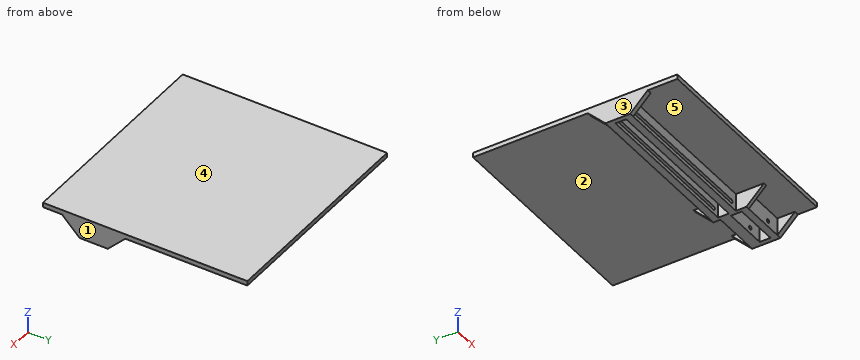
```python
from build123d import *

# Parameters (mm, degrees)
SKETCH_1_W          = 185
SKETCH_1_H          = 175
EXTRUDE_1_DEPTH     = 4
SKETCH_2_W          = 140
SKETCH_2_H          = 6
EXTRUDE_2_DEPTH     = 15
CUT_EXTRUDE_1_REACH = 210.987
SKETCH_4_W          = 45
SKETCH_4_H          = 9
SKETCH_4_H_2        = 6
EXTRUDE_5_DEPTH     = 15
SKETCH_7_W          = 185
SKETCH_7_H          = 4
EXTRUDE_6_DEPTH     = 40
SKETCH_6_W          = 185
SKETCH_6_H          = 4
CUT_EXTRUDE_3_DEPTH = 40
CUT_EXTRUDE_START   = -24.2
SKETCH_5_R          = 1.6
CUT_EXTRUDE_2_DEPTH = 24.2
EXTRUDE_7_DEPTH     = 3
EXTRUDE_8_DEPTH     = 4
EXTRUDE_9_DEPTH     = 4


with BuildPart() as part:
    # Sketch 1 → Extrude 1 (new body)
    with BuildSketch(Plane.XY):
        with Locations((21.366509782, 20.973731884)):
            Rectangle(SKETCH_1_W, SKETCH_1_H)
    extrude(amount=EXTRUDE_1_DEPTH)

    # Sketch 2 → Extrude 2 (add)
    with BuildSketch(Plane(origin=(0, 0, 0), x_dir=(-1, 0, 0), z_dir=(0, 0, -1))):
        with Locations((1.133490218, -63.126268116)):
            Rectangle(SKETCH_2_W, SKETCH_2_H)
        with Locations((1.133490218, -47.926268116)):
            Rectangle(SKETCH_2_W, SKETCH_2_H)
    extrude(amount=EXTRUDE_2_DEPTH)

    # Cut-Extrude 1: up to this face of the body (flat: up to its plane)
    cut_extrude_1_end = Plane(part.part.faces().sort_by_distance((-1.133490218, -44.926268116, -7.5))[0])
    # Sketch 3 → Cut-Extrude 1 (cut, up to the picked face)
    with BuildSketch(Plane.XZ.offset(66.126268116), mode=Mode.PRIVATE) as cut_extrude_1_sk1:
        with BuildLine():
            Line((-65.133490218, -8.4), (62.866509782, -8.4))
            ThreePointArc((62.866509782, -8.4), (64.466509782, -10), (62.866509782, -11.6))
            Line((62.866509782, -11.6), (-65.133490218, -11.6))
            ThreePointArc((-65.133490218, -11.6), (-66.733490218, -10), (-65.133490218, -8.4))
        make_face()
    cut_extrude_1_tool1 = split(extrude(cut_extrude_1_sk1.sketch, amount=-CUT_EXTRUDE_1_REACH, mode=Mode.PRIVATE), bisect_by=cut_extrude_1_end, keep=Keep.BOTH, mode=Mode.PRIVATE)
    add(cut_extrude_1_tool1.solids().sort_by(Axis((-1.13349, -66.126268, -10), (0, 1, 0)))[0], mode=Mode.SUBTRACT)

    # Sketch 4 → Extrude 5 (add)
    with BuildSketch(Plane(origin=(0, 0, 0), x_dir=(-1, 0, 0), z_dir=(0, 0, -1))):
        with Locations((-91.366509782, -55.526268116)):
            Rectangle(SKETCH_4_W, SKETCH_4_H)
        with Locations((-91.366509782, -72.226268116)):
            Rectangle(SKETCH_4_W, SKETCH_4_H_2)
    extrude(amount=EXTRUDE_5_DEPTH)


with BuildPart() as extrude_5_piece_1:
    # of the separate pieces the step leaves, piece 1, a body of its own (extrude_5_pieces)
    add(part.part.solids().sort_by_distance((-71.133490218, 108.473731884, 0))[0])

    # Sketch 7 → Extrude 6 (add)
    with BuildSketch(Plane.XZ.offset(66.526268116)):
        with Locations((21.366509782, 2)):
            Rectangle(SKETCH_7_W, SKETCH_7_H)
    extrude(amount=EXTRUDE_6_DEPTH)

    # Sketch 6 → Cut-Extrude 3 (cut)
    with BuildSketch(Plane(origin=(0, 108.473731884, 0), x_dir=(1, 0, 0), z_dir=(0, 1, 0))):
        with Locations((21.366509782, -2)):
            Rectangle(SKETCH_6_W, SKETCH_6_H)
    extrude(amount=-CUT_EXTRUDE_3_DEPTH, mode=Mode.SUBTRACT)


with BuildPart() as extrude_5_piece_2:
    # of the separate pieces the step leaves, piece 2, a body of its own (extrude_5_pieces)
    add(part.part.solids().sort_by_distance((68.866509782, -69.226268116, 0))[0])


with BuildPart() as cut_extrude_2_tool:
    # Sketch 5 → Cut-Extrude 2 (new body)
    with BuildSketch(Plane.XZ.offset(75.226268116).offset(CUT_EXTRUDE_START)):
        with Locations(Location((97.366509782, -10, 0), (0, 0, 270))):
            Circle(SKETCH_5_R)
    extrude(amount=CUT_EXTRUDE_2_DEPTH)


with BuildPart() as extrude_5_piece_1_1:
    add(extrude_5_piece_1.part)

    # Cut-Extrude 2: cut by cut_extrude_2_tool
    add(cut_extrude_2_tool.part, mode=Mode.SUBTRACT)



with BuildPart() as extrude_5_piece_2_1:
    add(extrude_5_piece_2.part)

    # Cut-Extrude 2: cut by cut_extrude_2_tool
    add(cut_extrude_2_tool.part, mode=Mode.SUBTRACT)


with BuildPart() as extrude_5_piece_1_2:
    add(extrude_5_piece_1_1.part)

    add(extrude_5_piece_2_1.part)  # Extrude 7 merges Extrude 5 piece 2
    # Sketch 8 → Extrude 7 (add)
    with BuildSketch(Plane(origin=(68.866509782, 0, 0), x_dir=(0, 0, -1), z_dir=(1, 0, 0))):
        Polygon((15, -44.926268116), (15, -75.226268116), (0, -90.226268116), (0, -29.926268116), align=None)
    extrude(amount=EXTRUDE_7_DEPTH)

    # Sketch 9 → Extrude 8 (add)
    with BuildSketch(Plane(origin=(113.866509782, 0, 0), x_dir=(0, 0, -1), z_dir=(1, 0, 0))):
        Polygon((15, -51.026268116), (15, -75.226268116), (0, -90.226268116), (0, -36.026268116), align=None)
    extrude(amount=-EXTRUDE_8_DEPTH)

    # Sketch 11 → Extrude 9 (add)
    with BuildSketch(Plane.ZY.offset(71.133490218)):
        Polygon((-15, -66.126268116), (-15, -44.926268116), (0, -29.926268116), (0, -81.126268116), align=None)
    extrude(amount=-EXTRUDE_9_DEPTH)


solid = extrude_5_piece_1_2.part
```
Verification items for the finished model (mm, model axes). Face numbers are marked on the shaded views. A direction names the side the tool comes from. Give positions to 0.01 mm unless a question says otherwise; leave off trailing zeros. Write each loop counter-clockwise with the first axis right and the second up, starting at its lowest first coordinate (ties: lowest second). Pieces come first, ordered by that corner, then holes. Notation, with made-up numbers: (84, 5.25) - (127, 5.25) arc R21 cw to (127, 9.25) - close; hole circle Ø11 at (2, 63.25). An arc over 180 degrees is marked (long way). Put each result on its own line as item: value.
Q1. Set-up check for the marked faces 1 and 2: record each of +Z, -Z, +X, -X, +Y, -Y from which the full face is reachable in a straight line by a thin tool's end or side.
Result:
face 1: +Z, -Z, +X, +Y, -Y
face 2: -Z, +Y
Q2. Section check B-B on z = -2.75. Record the cut outline in (x, y), and give its area (3 significant figures).
Result:
outline: (-71.13, -78.38) - (-67.13, -78.38) - (-67.13, -66.13) - (68.87, -66.13) - (68.87, -87.48) - (71.87, -87.48) - (71.87, -75.23) - (109.87, -75.23) - (109.87, -87.48) - (113.87, -87.48) - (113.87, -38.78) - (109.87, -38.78) - (109.87, -51.03) - (71.87, -51.03) - (71.87, -32.68) - (68.87, -32.68) - (68.87, -44.93) - (-67.13, -44.93) - (-67.13, -32.68) - (-71.13, -32.68) - close; hole (-67.13, -60.13) - (68.87, -60.13) - (68.87, -50.93) - (-67.13, -50.93) - close; hole (71.87, -69.23) - (109.87, -69.23) - (109.87, -60.03) - (71.87, -60.03) - close
area: 2,740 mm2
Q3. Scan lines: probe 1 along Y at (x, z) = (48, -5); probe 2 along X at (y, z) = (-72.9, -10); probe 3 along Z at (x, y) = (97.5, -13.5). Record each from-to range of solid material in increasing order. Write a range as from..to.
Result:
probe 1: -66.13..-60.13, -50.93..-44.93
probe 2: 68.87..95.77, 98.97..113.87
probe 3: 0..4
Q4. Section check A-A on x = -33.5. Record the cut outline in (y, z), and give its area (3 significant figures).
Result:
outline: (-106.53, 0) - (-66.13, 0) - (-66.13, -8.4) - (-60.13, -8.4) - (-60.13, 0) - (-50.93, 0) - (-50.93, -8.4) - (-44.93, -8.4) - (-44.93, 0) - (68.47, 0) - (68.47, 4) - (-106.53, 4) - close; (-66.13, -15) - (-60.13, -15) - (-60.13, -11.6) - (-66.13, -11.6) - close; (-50.93, -15) - (-44.93, -15) - (-44.93, -11.6) - (-50.93, -11.6) - close
area: 842 mm2
Q5. Depth check by flat-ended pin: P1, Ø6, axis at x = 36.5, y = -31.5, coming from the -Z side; P2, Ø4.5, axis at x = 92, z = -6.5, coming from the +Y side; P3, Ø4.5, axis at x = -7, z = -4.5, coming from the -Y side. Enter the tip coordinate at first touch or a pass-through.
Result:
P1: z = 0
P2: y = -51.03
P3: y = -66.13
Q6. Section check C-C on y = -25.5. Record the cut outline in (x, z).
Result:
outline: (-71.13, 0) - (113.87, 0) - (113.87, 4) - (-71.13, 4) - close
Q7. Mould release check, pull along X, two halves, no side actions. Record for the marked faces 3, 4 and 5: released by +X, released by -X, zero draft, split by the parting line, or undercut.
Result:
face 3: released by -X
face 4: zero draft
face 5: undercut
